For this review, take the finished solid that the model builds, in its own axes (mm). A direction names the side the tool comes from. Round coordinates to 2 decimals unless told otherwise and drop trailing zeros. Loops run counter-clockwise (first coordinate to the right, second up) from the corner with the lowest first, then second, coordinate; pieces in that order, holes last.
1. To check wall thickness, follow line 1 along Z through (x, y) = (0, -65); line 2 along X through (y, z) = (-9.5, 42.5); line 3 along Y through (x, z) = (8.5, 40.5). State the ranges of each line that lie inside material, in increasing order.
2. Consider section C-C on x = -1.5. State how many separate pieces and enclosed holes the cut face has, then the cut area to 3 significant figures.
3. Draft analysis for pull direction Y (two halves, no side actions). For faces 1 (the flat face through (0, 0, 47)), 2 (the flat face through (-6, -53, 95)), 3 (the cylindrical face through (4, -102, 12)), state which applies: released by +Y, released by -Y, zero draft, split by the parting line, or undercut.
4. Consider section A-A on y = -65. State the section outline as (x, z) points, then the cut area to 3 significant figures.
5. Tool access review of faces 4 (the cylindrical face through (8.57, -17.65, 41.85)), 5 (the cylindrical face through (13.483, -9.93, 42.24)), 6 (the flat face through (11, -5, 47)), 7 (the flat face through (12.5, -66, 39)): name each direction out of +Z, -Z, +X, -X, +Y, -Y from which nothing blocks a thin tool from reaching the whole face with its end or side.
6. Consider section B-B on z = 89. State the section outline as (x, y) points.
7. Consider section D-D on z = 72.5. State the section outline as (x, y) points, then the cut area to 3 significant figures.
8. Clearance check with flat-ended pins moving along their axes: pin 1 Ø10.5 at (y, z) = (-92, 72.5) entering from +X; pin 2 Ø2.5 at (x, z) = (11.5, 42.5) entering from +Y; pin 3 Ø1.5 at (y, z) = (-3.5, 41.5) entering from +X. State where each tip first meets the part, or that it passes through.
from build123d import *

# Parameters (mm, degrees)
BOSS_EXTRUDE1_DEPTH         = 95
SKETCH17_W                  = 95
SKETCH17_H                  = 105
BOSS_EXTRUDE3_DEPTH         = 7.5
SKETCH18_R                  = 7.5
CUT_EXTRUDE3_DEPTH          = 143.390308659
ESQUISSE1_R                 = 2
ENL_V_MAT_EXTRU_1_DEPTH     = 144.374509589
ESQUISSE3_R                 = 2
ENL_V_MAT_EXTRU_3_DEPTH     = 144.374509589
ESQUISSE4_R                 = 7.5
ESQUISSE4_R_2               = 10.5
ENL_V_MAT_EXTRU_4_DEPTH     = 143.390308659
ESQUISSE5_R                 = 4
ENL_V_MAT_EXTRU_15CNC_DEPTH = 144.374509589
ESQUISSE6_R                 = 1.5
ENL_V_MAT_EXTRU_19_DEPTH    = 144.374509589
ESQUISSE8_R                 = 2
ENL_V_MAT_EXTRU_20_DEPTH    = 15
ENL_V_START                 = -10
ESQUISSE8_3_R               = 3
ESQUISSE8_3_R_2             = 2
ENL_V_MAT_EXTRU_21_DEPTH    = 10
ESQUISSE9_R                 = 2.5
ENL_V_MAT_EXTRU_22_DEPTH    = 2.5


with BuildPart() as part:
    # Sketch1 → Boss-Extrude1 (new body)
    with BuildSketch(Plane.XY):
        Polygon((0, 0), (8, 0), (8, -5), (15, -5), (15, -9.75), (15, -24.75), (15, -43.75), (7, -43.75), (7, -53.25), (15, -53.25), (15, -60.75), (15, -105), (0, -105), align=None)
    extrude(amount=BOSS_EXTRUDE1_DEPTH)

    # Sketch17 → Boss-Extrude3 (add)
    with BuildSketch(Plane.ZY):
        with Locations((47.5, -52.5)):
            Rectangle(SKETCH17_W, SKETCH17_H)
    extrude(amount=BOSS_EXTRUDE3_DEPTH)

    # Sketch18 → Cut-Extrude3 (cut, through all)
    with BuildSketch(Plane.XY.offset(95)):
        with Locations((-6, -27)):
            Circle(SKETCH18_R)
        with Locations((-6, -78)):
            Circle(SKETCH18_R)
    extrude(amount=-CUT_EXTRUDE3_DEPTH, mode=Mode.SUBTRACT)

    # Esquisse1 → Enl_v. mat.-Extru.1 (cut, through all)
    with BuildSketch(Plane(origin=(15, 0, 0), x_dir=(0, 0, -1), z_dir=(1, 0, 0))):
        with Locations((-83, -100)):
            Circle(ESQUISSE1_R)
        with Locations(Location((-12, -100, 0), (0, 0, 180))):
            Circle(ESQUISSE1_R)
    extrude(amount=-ENL_V_MAT_EXTRU_1_DEPTH, mode=Mode.SUBTRACT)

    # Esquisse3 → Enl_v. mat.-Extru.3 (cut, through all)
    with BuildSketch(Plane(origin=(15, 0, 0), x_dir=(0, 0, -1), z_dir=(1, 0, 0))):
        with Locations((-6, -39.5)):
            Circle(ESQUISSE3_R)
        with Locations((-89, -39.5)):
            Circle(ESQUISSE3_R)
    extrude(amount=-ENL_V_MAT_EXTRU_3_DEPTH, mode=Mode.SUBTRACT)

    # Esquisse4 → Enl_v. mat.-Extru.4 (cut, through all)
    with BuildSketch(Plane(origin=(0, 0, 0), x_dir=(-1, 0, 0), z_dir=(0, 0, -1))):
        with Locations((-12, -78)):
            Circle(ESQUISSE4_R)
        with Locations((-12, -27)):
            Circle(ESQUISSE4_R)
        with Locations((-5, -52.5)):
            Circle(ESQUISSE4_R_2)
    extrude(amount=-ENL_V_MAT_EXTRU_4_DEPTH, mode=Mode.SUBTRACT)

    # Esquisse5 → Enl_v. mat.-Extru.15CNC (cut, through all)
    with BuildSketch(Plane(origin=(-7.5, 0, 0), x_dir=(0, 0, -1), z_dir=(1, 0, 0))):
        with Locations((-15, -10)):
            Circle(ESQUISSE5_R)
        with Locations((-80, -10)):
            Circle(ESQUISSE5_R)
        with Locations((-22.5, -92)):
            Circle(ESQUISSE5_R)
        with Locations(Location((-72.5, -92, 0), (0, 0, 180))):
            Circle(ESQUISSE5_R)
    extrude(amount=ENL_V_MAT_EXTRU_15CNC_DEPTH, mode=Mode.SUBTRACT)

    # Esquisse6 → Enl_v. mat.-Extru.19 (cut, through all)
    with BuildSketch(Plane(origin=(15, 0, 0), x_dir=(0, 0, -1), z_dir=(1, 0, 0))):
        with Locations((-32.5, -10)):
            Circle(ESQUISSE6_R)
        with Locations((-63.5, -10)):
            Circle(ESQUISSE6_R)
        with Locations((-63.5, -41)):
            Circle(ESQUISSE6_R)
        with Locations((-32.5, -41)):
            Circle(ESQUISSE6_R)
        with Locations((-40.5, -65)):
            Circle(ESQUISSE6_R)
        with Locations((-63.5, -65)):
            Circle(ESQUISSE6_R)
    extrude(amount=-ENL_V_MAT_EXTRU_19_DEPTH, mode=Mode.SUBTRACT)

    # Esquisse8 → Enl_v. mat.-Extru.20 (cut)
    with BuildSketch(Plane(origin=(0, -5, 0), x_dir=(1, 0, 0), z_dir=(0, 1, 0))):
        with Locations(Location((11.5, -42.5, 0), (0, 0, 270))):
            Circle(ESQUISSE8_R)
        with Locations(Location((11.5, -52.5, 0), (0, 0, 270))):
            Circle(ESQUISSE8_R)
    extrude(amount=-ENL_V_MAT_EXTRU_20_DEPTH, mode=Mode.SUBTRACT)

    # Esquisse8_3 → Enl_v. mat.-Extru.21 (cut)
    # profile 1 of 2: a face of its own
    with BuildSketch(Plane(origin=(0, -5, 0), x_dir=(1, 0, 0), z_dir=(0, 1, 0)).offset(ENL_V_START)):
        with Locations(Location((11.5, -42.5, 0), (0, 0, 270))):
            Circle(ESQUISSE8_3_R)
        with Locations(Location((11.5, -42.5, 0), (0, 0, 270))):
            Circle(ESQUISSE8_3_R_2, mode=Mode.SUBTRACT)
    # profile 2 of 2: a face of its own
    with BuildSketch(Plane(origin=(0, -5, 0), x_dir=(1, 0, 0), z_dir=(0, 1, 0)).offset(ENL_V_START)):
        with Locations(Location((11.5, -52.5, 0), (0, 0, 270))):
            Circle(ESQUISSE8_3_R)
        with Locations(Location((11.5, -52.5, 0), (0, 0, 270))):
            Circle(ESQUISSE8_3_R_2, mode=Mode.SUBTRACT)
    extrude(amount=-ENL_V_MAT_EXTRU_21_DEPTH, mode=Mode.SUBTRACT)

    # Esquisse9 → Enl_v. mat.-Extru.22 (cut)
    with BuildSketch(Plane(origin=(15, 0, 0), x_dir=(0, 0, -1), z_dir=(1, 0, 0))):
        with Locations((-40.5, -65)):
            Circle(ESQUISSE9_R)
        with Locations((-63.5, -65)):
            Circle(ESQUISSE9_R)
    extrude(amount=-ENL_V_MAT_EXTRU_22_DEPTH, mode=Mode.SUBTRACT)


solid = part.part
Resolved:
1. line 1: z = 0 to 39, 42 to 62, 65 to 95
1. line 2: x = -7.5 to 9.5, 13.5 to 15
1. line 3: y = -105 to -84.63, -71.37 to -66.5, -63.5 to -62.4, -42.6 to -33.63, -20.37 to -5
2. separate pieces: 4
2. enclosed holes: 14
2. area: 5,830 mm2
3. face 1: released by +Y
3. face 2: zero draft
3. face 3: undercut
4. outline: (-7.5, 0) - (15, 0) - (15, 38) - (12.5, 38) - (12.5, 39) - (-7.5, 39) - close; (-7.5, 42) - (12.5, 42) - (12.5, 43) - (15, 43) - (15, 61) - (12.5, 61) - (12.5, 62) - (-7.5, 62) - close; (-7.5, 65) - (12.5, 65) - (12.5, 66) - (15, 66) - (15, 95) - (-7.5, 95) - close
4. area: 1,990 mm2
5. face 4: none
5. face 5: +Y
5. face 6: +Z, -Z, +X, +Y
5. face 7: +X
6. outline: (-7.5, -105) - (15, -105) - (15, -84.87) arc R7.5 cw (long way) to (15, -71.13) - (15, -55.7) arc R10.5 cw (long way) to (10.8, -43.75) - (15, -43.75) - (15, -41.5) - (-7.5, -41.5) - (-7.5, -70.65) arc R7.5 cw (long way) to (-7.5, -85.35) - close; (-7.5, -37.5) - (15, -37.5) - (15, -33.87) arc R7.5 cw (long way) to (15, -20.13) - (15, -5) - (8, -5) - (8, 0) - (-7.5, 0) - (-7.5, -19.65) arc R7.5 cw (long way) to (-7.5, -34.35) - close
7. outline: (-7.5, -105) - (15, -105) - (15, -96) - (-7.5, -96) - close; (-7.5, -88) - (15, -88) - (15, -84.87) arc R7.5 cw (long way) to (15, -71.13) - (15, -55.7) arc R10.5 cw (long way) to (10.8, -43.75) - (15, -43.75) - (15, -33.87) arc R7.5 cw (long way) to (15, -20.13) - (15, -5) - (8, -5) - (8, 0) - (-7.5, 0) - (-7.5, -19.65) arc R7.5 cw (long way) to (-7.5, -34.35) - (-7.5, -70.65) arc R7.5 cw (long way) to (-7.5, -85.35) - close
7. area: 1,310 mm2
8. pin 1: stops at x = 15
8. pin 2: stops at y = -34.29
8. pin 3: stops at x = 8
